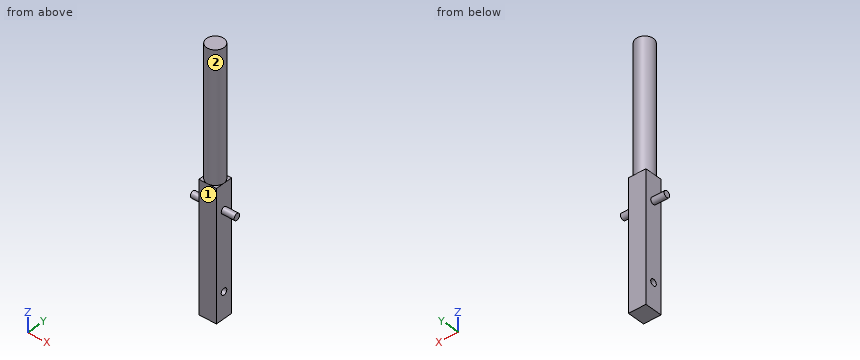
from build123d import *

# Parameters (mm, degrees)
F0_W          = 8.636
F0_H          = 8.636
F1_DEPTH      = 63.5
F2_R          = 4.318
F3_DEPTH      = 63.5
F4_R          = 1.5875
F5_DEPTH      = 25.4
F6_R          = 1.5875
F7_DEPTH      = 6.35
F7_DEPTH_BACK = 15.24


with BuildPart() as f1:
    # F0 (on Top) → F1 (new body)
    with BuildSketch(Plane.XY):
        Rectangle(F0_W, F0_H)
    extrude(amount=F1_DEPTH)

    # F2 (on face) → F3 (join)
    with BuildSketch(Plane.XY.offset(63.5)):
        Circle(F2_R)
    extrude(amount=F3_DEPTH)

    # F4 (on face) → F5 (cut)
    with BuildSketch(Plane.YZ.offset(4.318)):
        with Locations((0, 12.7)):
            Circle(F4_R)
    extrude(amount=-F5_DEPTH, mode=Mode.SUBTRACT)

    # F6 (on face) → F7 (join, two sides)
    with BuildSketch(Plane.YZ.offset(4.318)) as f7_sk:
        with Locations((0, 50.8)):
            Circle(F6_R)
    extrude(amount=F7_DEPTH)
    extrude(f7_sk.sketch, amount=-F7_DEPTH_BACK)


solid = f1.part
Model file for the job. Use its own axes, mm. Face numbers are marked on the shaded views. A direction names the side the tool comes from. Give positions to 0.01 mm unless a question says otherwise; leave off trailing zeros. Loops run counter-clockwise (first coordinate to the right, second up) from the corner with the lowest first, then second, coordinate; pieces in that order, holes last. Notation, with made-up numbers: (-18.5, -1) -> (40.5, -1) arc R30 ccw to (40.5, 38) -> close; hole circle Ø2 at (-31.5, 74.25). An arc over 180 degrees is marked (long way). Use a Markdown table: item, result. Add a question column.
(1) Slice it at D-D on z = 94.5. List the corners of the cut face in (x, y), and give its area (3 significant figures).
(2) Tool access for the marked faces 1 and 2: list every direction of +Z, -Z, +X, -X, +Y, -Y with a clear straight run to the whole face (end or side of a thin tool).
(3) Drop flat-ended pins along their axis: pin 1 Ø2 at (x, z) = (6.5, 14.5) entering from -Y; pin 2 Ø4 at (y, z) = (2.5, 45) entering from +X; pin 3 Ø5 at (y, z) = (-1.5, 87.5) entering from -X. Give the stop position or say it passes through.
(4) Wall check: line 1 along Z through (x, y) = (0.5, 0); line 2 along X through (y, z) = (2, 5.5); line 3 along Z through (x, y) = (-1.75, 0.75). Give the ranges that are in metal, low to high.
(5) Slice it at A-A on z = 50.8. List the corners of the cut face in (x, y), and give its area (3 significant figures).
(6) Slice it at B-B on y = 2.75. List the corners of the cut face in (x, z).
Filled sheet:
| question | item | result |
|---|---|---|
| 1 | outline | circle Ø8.64 at (0, 0) |
| 1 | area | 58.6 mm2 |
| 2 | face 1 | +Z, -Z, +X, -X, -Y |
| 2 | face 2 | +Z |
| 3 | pin 1 | through |
| 3 | pin 2 | x = 4.32 |
| 3 | pin 3 | x = -4.32 |
| 4 | line 1 | 0 to 11.11, 14.29 to 127 |
| 4 | line 2 | -4.32 to 4.32 |
| 4 | line 3 | 0 to 11.3, 14.1 to 127 |
| 5 | outline | (-10.92, -1.59) -> (-4.32, -1.59) -> (-4.32, -4.32) -> (4.32, -4.32) -> (4.32, -1.59) -> (10.67, -1.59) -> (10.67, 1.59) -> (4.32, 1.59) -> (4.32, 4.32) -> (-4.32, 4.32) -> (-4.32, 1.59) -> (-10.92, 1.59) -> close |
| 5 | area | 116 mm2 |
| 6 | outline | (-4.32, 0) -> (4.32, 0) -> (4.32, 63.5) -> (3.33, 63.5) -> (3.33, 127) -> (-3.33, 127) -> (-3.33, 63.5) -> (-4.32, 63.5) -> close |
